```python
from build123d import *

# Parameters (mm, degrees)
SKETCH1_R          = 15.6591
MOTOR_DEPTH        = 21.4122
SKETCH3_R          = 18.2245
GEARBOX_DEPTH      = 17.7292
SKETCH4_R          = 5.8801
PROTRUSION_DEPTH   = 4.6736
SKETCH5_R          = 2.921
SHAFT_DEPTH        = 18.4404
SKETCH6_R          = 1.27
SCREW_HOLES_DEPTH  = 9.3472
SKETCH7_R          = 4.4577
NUB_DEPTH          = 2.921
CUT_EXTRUDE1_DEPTH = 11.43


with BuildPart() as part:
    # Sketch1 → motor (new body)
    with BuildSketch(Plane.XY):
        Circle(SKETCH1_R)
    extrude(amount=MOTOR_DEPTH)

    # Sketch3 → gearbox (add)
    with BuildSketch(Plane.XY.offset(21.4122)):
        Circle(SKETCH3_R)
    extrude(amount=GEARBOX_DEPTH)

    # Sketch4 → protrusion (add)
    with BuildSketch(Plane.XY.offset(39.1414)):
        with Locations((0, -6.8834)):
            Circle(SKETCH4_R)
    extrude(amount=PROTRUSION_DEPTH)

    # Sketch5 → shaft (add)
    with BuildSketch(Plane.XY.offset(43.815)):
        with Locations((0, -6.8834)):
            Circle(SKETCH5_R)
    extrude(amount=SHAFT_DEPTH)

    # Sketch6 → screw holes (cut)
    with BuildSketch(Plane.XY.offset(39.1414)):
        with Locations((15.24, 0)):
            Circle(SKETCH6_R)
        with Locations((-15.24, 0)):
            Circle(SKETCH6_R)
        with Locations((-7.62, -13.198227096)):
            Circle(SKETCH6_R)
        with Locations((-7.61999995, 13.198227183)):
            Circle(SKETCH6_R)
    extrude(amount=-SCREW_HOLES_DEPTH, mode=Mode.SUBTRACT)

    # Sketch7 → nub (add)
    with BuildSketch(Plane(origin=(0, 0, 0), x_dir=(-1, 0, 0), z_dir=(0, 0, -1))):
        with Locations(Location((0, 0, 0), (0, 0, 180))):  # turned: the seam where the file's is
            Circle(SKETCH7_R)
    extrude(amount=NUB_DEPTH)

    # Sketch8 → Cut-Extrude1 (cut)
    with BuildSketch(Plane.XY.offset(62.2554)):
        with BuildLine():
            Line((1.260039062, -4.24815), (-1.260039062, -4.24815))
            ThreePointArc((-1.260039062, -4.24815), (0, -3.9624), (1.260039062, -4.24815))
        make_face()
    extrude(amount=-CUT_EXTRUDE1_DEPTH, mode=Mode.SUBTRACT)


solid = part.part
```
Work out the finished part from the listing and answer in its coordinate system (mm). A direction names the side the tool comes from. Give positions to 0.01 mm unless a question says otherwise; leave off trailing zeros. Write each loop counter-clockwise with the first axis right and the second up, starting at its lowest first coordinate (ties: lowest second). Pieces come first, ordered by that corner, then holes. Notation, with made-up numbers: (45.5, 51.5) -> (85.5, 51.5) arc R30 cw to (85.5, 83.5) -> close; hole circle Ø8 at (57.25, 49.25). An arc over 180 degrees is marked (long way). Write each question's results on one line, items separated by ' | '.
1. Each of these flat-tipped pins is pushed along its axis until it touches: pin 1 Ø3.5 at (x, y) = (-15.24, 0) entering from +Z; pin 2 Ø3 at (x, y) = (15.24, 0) entering from -Z; pin 3 Ø3 at (x, z) = (-0.5, 57) entering from +Y; pin 4 Ø3 at (x, y) = (-14, -14.5) entering from -Z. Where does it stop, or does it pass through?
Data:
pin 1: z = 39.14 | pin 2: z = 0 | pin 3: y = -4.25 | pin 4: through
2. Find section B-B on y = 8. Determine the outline of the cut face in (x, z).
Data:
outline: (-16.37, 21.41) -> (-13.46, 21.41) -> (-13.46, 0) -> (13.46, 0) -> (13.46, 21.41) -> (16.37, 21.41) -> (16.37, 39.14) -> (-16.37, 39.14) -> close
3. Straight lines are drawn through the part: L1, parallel to Y at x = -7.62, z = 33.5 (3 decimals); L2, parallel to Z at x = 1.5, y = 3; L3, parallel to Z at x = -12, y = -5. For each, find the intervals that lie inside material, in ascending order.
Data:
L1: -16.555 to -14.468, -11.928 to 11.928, 14.468 to 16.555 | L2: -2.92 to 39.14 | L3: 0 to 39.14
4. Find section D-D on y = 0. Determine the outline of the cut face in (x, z).
Data:
outline: (-18.22, 21.41) -> (-15.66, 21.41) -> (-15.66, 0) -> (-4.46, 0) -> (-4.46, -2.92) -> (4.46, -2.92) -> (4.46, 0) -> (15.66, 0) -> (15.66, 21.41) -> (18.22, 21.41) -> (18.22, 39.14) -> (16.51, 39.14) -> (16.51, 29.79) -> (13.97, 29.79) -> (13.97, 39.14) -> (-13.97, 39.14) -> (-13.97, 29.79) -> (-16.51, 29.79) -> (-16.51, 39.14) -> (-18.22, 39.14) -> close
5. A tool of negligible diameter and unlimited length cuts with its end or side. For faces 5 (the flat face through (-15, 0, 29.794)), 6 (the flat face through (0, -4.248, 57)), 7 (the flat face through (0, 0, -2.921)), 8 (the cylindrical face through (-3.95, -17.79, 30.15)), 9 (the cylindrical face through (4.25, -1.34, -1.44)), from which of +Z, -Z, +X, -X, +Y, -Y can it reach the whole face along a straight path? Write none if from no direction.
Data:
face 5: +Z | face 6: +Z, +X, -X, +Y | face 7: -Z, +X, -X, +Y, -Y | face 8: +Z, -Z | face 9: -Z
6. Determine the mould class of faces 1 (the flat face through (-3, -8, 43.815)), 2 (the cylindrical face through (5.61, -5.12, 41.45)), 3 (the flat face through (-8, 13, 29.794)), 4 (the cylindrical face through (-16.176, 0.858, 34.533)) for opening direction Y: +Y half, -Y half, draft (parallel to the pull), parting line (faces both ways), or undercut.
Data:
face 1: draft | face 2: parting line | face 3: undercut | face 4: undercut
7. Find section C-C on z = 56. Determine the outline of the cut face in (x, y).
Data:
outline: (-1.26, -4.25) arc R2.92 ccw (long way) to (1.26, -4.25) -> close
